```python
from build123d import *

# Parameters (mm, degrees)
SKETCH_1_W          = 20
SKETCH_1_H          = 20
SKETCH_1_W_2        = 18
SKETCH_1_H_2        = 18
EXTRUDE_1_DEPTH     = 127
SKETCH_2_R          = 1.575
CUT_EXTRUDE_1_DEPTH = 131.111490653
SKETCH_3_R          = 1.6
CUT_EXTRUDE_2_DEPTH = 131.111490653


with BuildPart() as part:
    # 草图1 → 拉伸-薄壁1 (new body)
    with BuildSketch(Plane.XY):
        with Locations((10, -10)):
            Rectangle(SKETCH_1_W, SKETCH_1_H)
        with Locations((10, -10)):
            Rectangle(SKETCH_1_W_2, SKETCH_1_H_2, mode=Mode.SUBTRACT)
    extrude(amount=EXTRUDE_1_DEPTH)

    # 草图2 → 切除-拉伸1 (cut, through all)
    with BuildSketch(Plane.XZ.offset(20)):
        with Locations(Location((10, 11, 0), (0, 0, 270))):
            Circle(SKETCH_2_R)
        with Locations(Location((10, 31, 0), (0, 0, 270))):
            Circle(SKETCH_2_R)
        with Locations(Location((10, 51, 0), (0, 0, 270))):
            Circle(SKETCH_2_R)
        with Locations(Location((10, 71, 0), (0, 0, 270))):
            Circle(SKETCH_2_R)
        with Locations(Location((10, 91, 0), (0, 0, 270))):
            Circle(SKETCH_2_R)
        with Locations(Location((10, 111, 0), (0, 0, 270))):
            Circle(SKETCH_2_R)
        Polygon((10, 45.5), (5.669872981, 43), (5.669872981, 38), (10, 35.5), (14.330127019, 38), (14.330127019, 43), align=None)
        Polygon((10, 25.5), (5.669872981, 23), (5.669872981, 18), (10, 15.5), (14.330127019, 18), (14.330127019, 23), align=None)
        Polygon((10, 65.5), (5.669872981, 63), (5.669872981, 58), (10, 55.5), (14.330127019, 58), (14.330127019, 63), align=None)
        Polygon((10, 85.5), (5.669872981, 83), (5.669872981, 78), (10, 75.5), (14.330127019, 78), (14.330127019, 83), align=None)
        Polygon((10, 105.5), (5.669872981, 103), (5.669872981, 98), (10, 95.5), (14.330127019, 98), (14.330127019, 103), align=None)
    extrude(amount=-CUT_EXTRUDE_1_DEPTH, mode=Mode.SUBTRACT)

    # 草图3 → 切除-拉伸2 (cut, through all)
    with BuildSketch(Plane.ZY):
        with Locations(Location((122, -5, 0), (0, 0, 270))):
            Circle(SKETCH_3_R)
        with Locations(Location((122, -15, 0), (0, 0, 270))):
            Circle(SKETCH_3_R)
        with Locations(Location((112, -15, 0), (0, 0, 270))):
            Circle(SKETCH_3_R)
        with Locations(Location((112, -5, 0), (0, 0, 270))):
            Circle(SKETCH_3_R)
        with Locations(Location((97, -5, 0), (0, 0, 270))):
            Circle(SKETCH_3_R)
        with Locations(Location((97, -15, 0), (0, 0, 270))):
            Circle(SKETCH_3_R)
        with Locations(Location((87, -15, 0), (0, 0, 270))):
            Circle(SKETCH_3_R)
        with Locations(Location((87, -5, 0), (0, 0, 270))):
            Circle(SKETCH_3_R)
        with Locations(Location((72, -5, 0), (0, 0, 270))):
            Circle(SKETCH_3_R)
        with Locations(Location((72, -15, 0), (0, 0, 270))):
            Circle(SKETCH_3_R)
        with Locations(Location((62, -15, 0), (0, 0, 270))):
            Circle(SKETCH_3_R)
        with Locations(Location((62, -5, 0), (0, 0, 270))):
            Circle(SKETCH_3_R)
        with Locations(Location((47, -5, 0), (0, 0, 270))):
            Circle(SKETCH_3_R)
        with Locations(Location((47, -15, 0), (0, 0, 270))):
            Circle(SKETCH_3_R)
        with Locations(Location((37, -15, 0), (0, 0, 270))):
            Circle(SKETCH_3_R)
        with Locations(Location((37, -5, 0), (0, 0, 270))):
            Circle(SKETCH_3_R)
        with Locations(Location((22, -5, 0), (0, 0, 270))):
            Circle(SKETCH_3_R)
        with Locations(Location((22, -15, 0), (0, 0, 270))):
            Circle(SKETCH_3_R)
        with Locations(Location((12, -15, 0), (0, 0, 270))):
            Circle(SKETCH_3_R)
        with Locations(Location((12, -5, 0), (0, 0, 270))):
            Circle(SKETCH_3_R)
    extrude(amount=-CUT_EXTRUDE_2_DEPTH, mode=Mode.SUBTRACT)


solid = part.part
```
Input: part model. Units: mm. Frame: model coordinates. A direction names the side the tool comes from. Coordinates: 2 decimals unless noted, no trailing zeros. Order: outer loops, then holes, each group sorted by start corner. A loop starts at its lowest first (then second) coordinate and runs counter-clockwise, first axis right, second up. Notation, with made-up numbers: (23.25, -13.75) - (42.25, -13.75) arc R23 cw to (42.25, 20.25) - close; hole circle Ø5 at (14, -28.5). An arc over 180 degrees is marked (long way). Return JSON: item names as keys, results as strings.
Q1. Access query for faces 1 (the flat face through (19, -10, 63)), 2 (the flat face through (12.2, -19.51, 104.23)), 3 (the cylindrical face through (0.493, -14.792, 73.586)). Directions: +Z, -Z, +X, -X, +Y, -Y. A direction counts if a zero-diameter tool reaches every point of the face in a straight line with its end or side. Return the directions, or none.
The answers:
{"face 1": "+Z, -Z", "face 2": "+Y, -Y", "face 3": "+X, -X"}
Q2. Cut plane A-A (z = 31). Return loops of the section in (x, y) (3 decimals), then the cut area to 3 significant figures.
The answers:
{"outline": "(0, -20) - (8.425, -20) - (8.425, -19) - (1, -19) - (1, -1) - (8.425, -1) - (8.425, 0) - (0, 0) - close; (11.575, -20) - (20, -20) - (20, 0) - (11.575, 0) - (11.575, -1) - (19, -1) - (19, -19) - (11.575, -19) - close", "area": "69.7 mm2"}
Q3. Cut plane D-D (y = -14.75). State how many separate pieces and enclosed holes the cut face has, then the cut area to 3 significant figures.
The answers:
{"separate pieces": "22", "enclosed holes": "0", "area": "191 mm2"}
Q4. Cut plane C-C (y = -8.5). Return loops of the section in (x, z), then the cut area to 3 significant figures.
The answers:
{"outline": "(0, 0) - (1, 0) - (1, 127) - (0, 127) - close; (19, 0) - (20, 0) - (20, 127) - (19, 127) - close", "area": "254 mm2"}
Q5. Ray query, probe 1 along Y at (x, z) = (0.55, 122); probe 2 along X at (y, z) = (-9.5, 105); probe 3 along Y at (x, z) = (17.75, 39). Return the intervals inside material, ascending.
The answers:
{"probe 1": "y = -20 to -16.6, -13.4 to -6.6, -3.4 to 0", "probe 2": "x = 0 to 1, 19 to 20", "probe 3": "y = -20 to -19, -1 to 0"}
Q6. Cut plane B-B (x = 3). Return loops of the section in (y, z).
The answers:
{"outline": "(-20, 0) - (-19, 0) - (-19, 127) - (-20, 127) - close; (-1, 0) - (0, 0) - (0, 127) - (-1, 127) - close"}
Q7. Draft query along X for faces 4 (the flat face through (5, 0, 63)), 5 (the flat face through (7.8, -19.51, 96.77)). Return one class per face: +X half, -X half, draft (parallel to the pull), parting line (faces both ways), or undercut.
The answers:
{"face 4": "draft", "face 5": "undercut"}
Q8. First-contact query: pin 1 (1 mm diameter, centred on x = 11.5, z = 53, fed in from +Y); pin 2 (3 mm diameter, centred on x = 10, z = 71, fed in from -Y). Flat tips, straight axial feed; report the tip coordinate or a pass-through.
The answers:
{"pin 1": "stops at y = 0", "pin 2": "passes through"}
